The model under review builds one solid part; all positions refer to its coordinate system, in mm. A direction names the side the tool comes from. Coordinates: 2 decimals unless noted, no trailing zeros. Write each loop counter-clockwise with the first axis right and the second up, starting at its lowest first coordinate (ties: lowest second). Pieces come first, ordered by that corner, then holes. Notation, with made-up numbers: M 75.25,-29 L 88.25,-29 A12 ccw 88.25,-10 Z; hole C -17.75,69.5 d9. An arc over 180 degrees is marked long. Answer as CSV lines item,"result". Start each with the question number.
from build123d import *

# Parameters (mm, degrees)
EXTRUDE_1_DEPTH     = 26
SKETCH_3_W          = 20
SKETCH_3_H          = 20
CUT_EXTRUDE_1_DEPTH = 30
SKETCH_4_R          = 1.65
CUT_EXTRUDE_2_DEPTH = 69.713384893
SKETCH_4_3_R        = 4.15
SKETCH_4_3_R_2      = 1.65
CUT_EXTRUDE_3_DEPTH = 0.5
CUT_EXTRUDE_START   = -25.5
SKETCH_4_4_R        = 4.15
SKETCH_4_4_R_2      = 1.65
CUT_EXTRUDE_4_DEPTH = 0.5
SKETCH_5_R          = 2.1
CUT_EXTRUDE_5_DEPTH = 69.713384893
CUT_EXTRUDE_START_2 = -67
CUT_EXTRUDE_6_DEPTH = 67


with BuildPart() as part:
    # 草图2 → 凸台-拉伸1 (new body)
    with BuildSketch(Plane.XY):
        with BuildLine():
            Line((0, 0), (0, 30))
            ThreePointArc((0, 30), (13, 56.401219467), (26, 30))
            Line((26, 30), (26, 0))
            Line((26, 0), (0, 0))
        make_face()
    extrude(amount=EXTRUDE_1_DEPTH)

    # 草图3 → 切除-拉伸1 (cut)
    with BuildSketch(Plane.XZ):
        with Locations((13, 13)):
            Rectangle(SKETCH_3_W, SKETCH_3_H)
    extrude(amount=-CUT_EXTRUDE_1_DEPTH, mode=Mode.SUBTRACT)

    # 草图4 → 切除-拉伸2 (cut, through all)
    with BuildSketch(Plane.XY.offset(26)):
        with Locations((13, 40)):
            Circle(SKETCH_4_R)
    extrude(amount=-CUT_EXTRUDE_2_DEPTH, mode=Mode.SUBTRACT)

    # 草图4<3> → 切除-拉伸3 (cut)
    with BuildSketch(Plane.XY.offset(26)):
        with Locations((13, 40)):
            Circle(SKETCH_4_3_R)
        with Locations((13, 40)):
            Circle(SKETCH_4_3_R_2, mode=Mode.SUBTRACT)
    extrude(amount=-CUT_EXTRUDE_3_DEPTH, mode=Mode.SUBTRACT)

    # 草图4<4> → 切除-拉伸4 (cut)
    with BuildSketch(Plane.XY.offset(26).offset(CUT_EXTRUDE_START)):
        with Locations((13, 40)):
            Circle(SKETCH_4_4_R)
        with Locations((13, 40)):
            Circle(SKETCH_4_4_R_2, mode=Mode.SUBTRACT)
    extrude(amount=-CUT_EXTRUDE_4_DEPTH, mode=Mode.SUBTRACT)

    # 草图5 → 切除-拉伸5 (cut, through all)
    with BuildSketch(Plane.XY.offset(26)):
        with Locations((13, 22.5)):
            Circle(SKETCH_5_R)
        with Locations((13, 10)):
            Circle(SKETCH_5_R)
    extrude(amount=-CUT_EXTRUDE_5_DEPTH, mode=Mode.SUBTRACT)

    # 草图6 → 切除-拉伸6 (cut)
    with BuildSketch(Plane.XY.offset(26).offset(CUT_EXTRUDE_START_2)):
        with BuildLine():
            Line((0, 30), (0, 39.821933649))
            ThreePointArc((0, 39.821933649), (13, 53.001219467), (26, 39.821933649))
            Line((26, 39.821933649), (26, 30))
            ThreePointArc((26, 30), (13, 56.401219467), (0, 30))
        make_face()
    extrude(amount=CUT_EXTRUDE_6_DEPTH, mode=Mode.SUBTRACT)


solid = part.part
1) Take a section at C-C on y = 14. Give the boundary of the cut face in (x, z).
2) Take a section at A-A on y = 22.5. Give the boundary of the cut face in (x, z), and give its area (3 significant figures).
3) Take a section at D-D on x = 13. Give the number of separate pieces and of enclosed holes in the cut face, and give its area (3 significant figures).
4) Tool access review of faces 5 (the cylindrical face through (12.46, 44.115, 25.754)), 6 (the flat face through (13, 15, 23)), 7 (the cylindrical face through (12.46, 44.115, 0.254)): name each direction out of +Z, -Z, +X, -X, +Y, -Y from which nothing blocks a thin tool from reaching the whole face with its end or side.
5) Mouldability with a two-part tool opening along Z and no side actions: class faces 1 (the flat face through (25, 0, 13)), 2 (the flat face through (3, 15, 13)), 3 (the flat face through (13, 38, 0.5)), 4 (the flat face through (13, 38, 25.5)) as +Z half, -Z half, draft (parallel to the pull), parting line (faces both ways), or undercut.
6) To check wall thickness, follow line 1 (Z direction, x = 10.25, y = 24.5); line 2 (X direction, y = 38.5, z = 19.5). State the ranges of each line that lie inside material, in increasing order. Write a range as [from, to].
7) Clearance check with flat-ended pins moving along their axes: pin 1 Ø4 at (x, y) = (15, 39) entering from -Z; pin 2 Ø4 at (x, y) = (13.5, 38.5) entering from +Z; pin 3 Ø1 at (x, z) = (5.5, 7) entering from -Y; pin 4 Ø5.5 at (x, y) = (13, 40) entering from -Z. State where each tip first meets the part, or that it passes through.
Results:
1,outline,"M 0,0 L 26,0 L 26,26 L 0,26 Z; hole M 3,3 L 23,3 L 23,23 L 3,23 Z"
2,outline,"M 0,0 L 10.9,0 L 10.9,3 L 3,3 L 3,23 L 10.9,23 L 10.9,26 L 0,26 Z; M 15.1,0 L 26,0 L 26,26 L 15.1,26 L 15.1,23 L 23,23 L 23,3 L 15.1,3 Z"
2,area,"251 mm²"
3,separate pieces,"6"
3,enclosed holes,"0"
3,area,"637 mm²"
4,face 5,"+Z"
4,face 6,"-Y"
4,face 7,"-Z"
5,face 1,"draft"
5,face 2,"undercut"
5,face 3,"-Z half"
5,face 4,"+Z half"
6,line 1,"z = [0, 3], [23, 26]"
6,line 2,"x = [0, 12.31], [13.69, 26]"
7,pin 1,"stops at z = 0"
7,pin 2,"stops at z = 25.5"
7,pin 3,"stops at y = 30"
7,pin 4,"stops at z = 0.5"
